Verification items for the finished model (mm, model axes). A direction names the side the tool comes from. Give positions to 0.01 mm unless a question says otherwise; leave off trailing zeros. Loops run counter-clockwise (first coordinate to the right, second up) from the corner with the lowest first, then second, coordinate; pieces in that order, holes last. Notation, with made-up numbers: (5.25, 74.5) -> (43.25, 74.5) arc R23 cw to (43.25, 82.5) -> close; hole circle Ø9 at (9, 79.5). An arc over 180 degrees is marked (long way). Use one line per item in the form item = value. Start each with the question number.
from build123d import *

# Parameters (mm, degrees)
SKETCH1_W           = 150
SKETCH1_H           = 20
BOSS_EXTRUDE1_DEPTH = 10
BOSS_EXTRUDE2_DEPTH = 10
SKETCH7_W           = 150.099930891
SKETCH7_H           = 10
BOSS_EXTRUDE3_DEPTH = 23
SKETCH8_R           = 3
CUT_EXTRUDE4_DEPTH  = 46


with BuildPart() as part:
    # Sketch1 → Boss-Extrude1 (new, symmetric)
    with BuildSketch(Plane(origin=(0, 0, 0), x_dir=(1, 0, 0), z_dir=(0, 1, 0))):
        Rectangle(SKETCH1_W, SKETCH1_H)
    extrude(amount=BOSS_EXTRUDE1_DEPTH, both=True)

    # Sketch2 → Boss-Extrude2 (add, symmetric)
    with BuildSketch(Plane.XY):
        Polygon((-75, 10), (75, 10), (75, 41.883484251), align=None)
    extrude(amount=BOSS_EXTRUDE2_DEPTH, both=True)

    # Sketch7 → Boss-Extrude3 (add, symmetric)
    with BuildSketch(Plane.XY):
        with Locations((-0.049965445, -5)):
            Rectangle(SKETCH7_W, SKETCH7_H)
    extrude(amount=BOSS_EXTRUDE3_DEPTH, both=True)

    # Sketch8 → Cut-Extrude4 (cut)
    with BuildSketch(Plane(origin=(0, 0, 10), x_dir=(1, 0, 0), z_dir=(0, 1, 0))):
        with Locations(Location((-56.099930891, 26.5, 0), (0, 0, 180))):
            Circle(SKETCH8_R)
        with Locations(Location((56, 26.5, 0), (0, 0, 180))):
            Circle(SKETCH8_R)
        with Locations(Location((56, -6.5, 0), (0, 0, 180))):
            Circle(SKETCH8_R)
        with Locations(Location((-56.099930891, -6.5, 0), (0, 0, 180))):
            Circle(SKETCH8_R)
    extrude(amount=-CUT_EXTRUDE4_DEPTH, mode=Mode.SUBTRACT)


solid = part.part
Item 1: Sectioned sample at B-B, the plane x = 56. Enter the section's corners in (y, z), and give its area (3 significant figures).
Item 2: Tool access check on faces 1 (the flat face through (16, 17, -10)), 2 (the flat face through (-75, 5, 0)), 3 (the flat face through (16, 17, 10)). Record the directions out of +Z, -Z, +X, -X, +Y, -Y that give a thin tool (end or side, any length) a straight path to the whole face; none if there is none.
Item 3: Sectioned sample at C-C, the plane y = 7. Enter the section's corners in (x, z).
Item 4: Material ranges on line 1 (Z direction, x = 56, y = -5); line 2 (Y direction, x = -44, z = -13); line 3 (X direction, y = -2, z = -16), recorded low to high.
Item 5: Draft check along X on faces 4 (the flat face through (75, 10, 0)), 5 (the flat face through (-1, -5, 23)), 6 (the flat face through (-75.1, -5, 0)), 7 (the cylindrical face through (59, -4.9, 16.6)). Enter one of: +X half, -X half, draft (parallel to the pull), parting line (faces both ways), or undercut.
Item 6: Sectioned sample at D-D, the plane x = -0.5. Enter the section's corners in (y, z).
Item 7: Sectioned sample at A-A, the plane z = -16.5. Enter the section's corners in (x, y), and give its area (3 significant figures).
Item 8: Gauge pin test, flat ends, axial feed: pin 1 Ø1 at (x, y) = (56.5, 31) entering from +Z; pin 2 Ø8 at (x, z) = (56, 16.5) entering from +Y; pin 3 Ø5 at (x, z) = (-56.1, -16.5) entering from +Y; pin 4 Ø14 at (x, z) = (-37, 9.5) entering from +Y. Record the tip position at first contact, or that the pin passes through.
Outcome:
q1.outline = (-10, -23) -> (0, -23) -> (0, -19.5) -> (-10, -19.5) -> close; (-10, -13.5) -> (0, -13.5) -> (0, -10) -> (37.84, -10) -> (37.84, 10) -> (0, 10) -> (0, 13.5) -> (-10, 13.5) -> close; (-10, 19.5) -> (0, 19.5) -> (0, 23) -> (-10, 23) -> close
q1.area = 1,100 mm^2
q2.face_1 = -Z, +X, -X, +Y
q2.face_2 = +Z, -Z, -X, +Y
q2.face_3 = +Z, +X, -X, +Y
q3.outline = (-75, -10) -> (75, -10) -> (75, 10) -> (-75, 10) -> close
q4.line_1 = -23 to -19.5, -13.5 to 13.5, 19.5 to 23
q4.line_2 = -10 to 0
q4.line_3 = -75.1 to -59.06, -53.14 to 53.04, 58.96 to 75
q5.face_4 = +X half
q5.face_5 = draft
q5.face_6 = -X half
q5.face_7 = undercut
q6.outline = (-10, -23) -> (0, -23) -> (0, -10) -> (25.84, -10) -> (25.84, 10) -> (0, 10) -> (0, 23) -> (-10, 23) -> close
q7.outline = (-75.1, -10) -> (-59.1, -10) -> (-59.1, 0) -> (-75.1, 0) -> close; (-53.1, -10) -> (53, -10) -> (53, 0) -> (-53.1, 0) -> close; (59, -10) -> (75, -10) -> (75, 0) -> (59, 0) -> close
q7.area = 1,380 mm^2
q8.pin_1 = 10
q8.pin_2 = 0
q8.pin_3 = through
q8.pin_4 = 19.57
